For this review, take the finished solid that the model builds, in its own axes (mm). A direction names the side the tool comes from. Round coordinates to 2 decimals unless told otherwise and drop trailing zeros. Loops run counter-clockwise (first coordinate to the right, second up) from the corner with the lowest first, then second, coordinate; pieces in that order, holes last. Notation, with made-up numbers: (11, 36.25) -> (60, 36.25) arc R27 ccw to (60, 62.25) -> close; hole circle Ø10 at (59, 45.25). An arc over 180 degrees is marked (long way). Write each question's results on one line, items separated by ' | '.
```python
from build123d import *

# Parameters (mm, degrees)
Y_KSEKLIK_EKSTR_ZYON1_DEPTH             = 19
IZIM2_W                                 = 40
IZIM2_H                                 = 40
Y_KSEKLIK_EKSTR_ZYON2_DEPTH             = 9
IZIM5_W                                 = 46
IZIM5_H                                 = 46
IZIM5_W_2                               = 40
IZIM5_H_2                               = 40
Y_KSEKLIK_EKSTR_ZYON3_DEPTH             = 9
Y_KSEKLIK_EKSTR_ZYON3_DIRECTION_2_REACH = 172.345
KES_EKSTR_ZYON1_DEPTH                   = 9
KES_EKSTR_ZYON1_DEPTH_BACK              = 9
IZIM7_W                                 = 15
IZIM7_H                                 = 15
IZIM8_R                                 = 3.25
KES_EKSTR_ZYON2_DEPTH                   = 163


with BuildPart() as part:
    # Çizim1 → Yükseklik-Ekstrüzyon1 (new body)
    with BuildSketch(Plane.XY):
        Polygon((0, 0), (0, 80), (133, 80), (133, 0), (138, 0), (138, 30), (142, 30), (142, 89), (-9, 89), (-9, 30), (-5, 30), (-5, 0), align=None)
    extrude(amount=Y_KSEKLIK_EKSTR_ZYON1_DEPTH)

    # Çizim2 → Yükseklik-Ekstrüzyon2 (add)
    with BuildSketch(Plane(origin=(0, 89, 0), x_dir=(1, 0, 0), z_dir=(0, 1, 0))):
        with Locations((66.5, -10.538159249)):
            Rectangle(IZIM2_W, IZIM2_H)
    extrude(amount=-Y_KSEKLIK_EKSTR_ZYON2_DEPTH)

    # Çizim5 → Yükseklik-Ekstrüzyon3 (add)
    with BuildSketch(Plane(origin=(0, 89, 0), x_dir=(1, 0, 0), z_dir=(0, 1, 0))):
        with Locations((66.5, -10.538159249)):
            Rectangle(IZIM5_W, IZIM5_H)
        with Locations((66.5, -10.538159249)):
            Rectangle(IZIM5_W_2, IZIM5_H_2, mode=Mode.SUBTRACT)
    extrude(amount=Y_KSEKLIK_EKSTR_ZYON3_DEPTH)

    # Yükseklik-Ekstrüzyon3 direction 2: up to this face of the body (flat: up to its plane)
    y_kseklik_ekstr_zyon3_direction_2_end = Plane(part.part.faces().sort_by_distance((66.5, 80, 9.993333768))[0])
    # Çizim5 → Yükseklik-Ekstrüzyon3 direction 2 (add, up to the picked face)
    with BuildSketch(Plane(origin=(0, 89, 0), x_dir=(1, 0, 0), z_dir=(0, 1, 0)), mode=Mode.PRIVATE) as y_kseklik_ekstr_zyon3_direction_2_sk1:
        with Locations((66.5, -10.538159249)):
            Rectangle(IZIM5_W, IZIM5_H)
        with Locations((66.5, -10.538159249)):
            Rectangle(IZIM5_W_2, IZIM5_H_2, mode=Mode.SUBTRACT)
    y_kseklik_ekstr_zyon3_direction_2_tool1 = split(extrude(y_kseklik_ekstr_zyon3_direction_2_sk1.sketch, amount=-Y_KSEKLIK_EKSTR_ZYON3_DIRECTION_2_REACH, mode=Mode.PRIVATE), bisect_by=y_kseklik_ekstr_zyon3_direction_2_end, keep=Keep.BOTH, mode=Mode.PRIVATE)
    add(y_kseklik_ekstr_zyon3_direction_2_tool1.solids().sort_by(Axis((66.5, 89, 32.887621), (0, -1, 0)))[0])

    # Çizim7 → Kes-Ekstrüzyon1 (cut, two sides: drawn at the far end of the back side and taken through both)
    with BuildSketch(Plane(origin=(0, 89, 0), x_dir=(1, 0, 0), z_dir=(0, 1, 0)).offset(-KES_EKSTR_ZYON1_DEPTH_BACK)):
        with Locations((66.5, -10.538159249)):
            Rectangle(IZIM7_W, IZIM7_H)
    extrude(amount=KES_EKSTR_ZYON1_DEPTH + KES_EKSTR_ZYON1_DEPTH_BACK, mode=Mode.SUBTRACT)

    # Çizim8 → Kes-Ekstrüzyon2 (cut)
    with BuildSketch(Plane(origin=(138, 0, 0), x_dir=(0, 0, -1), z_dir=(1, 0, 0))):
        with Locations((-9.5, 15)):
            Circle(IZIM8_R)
    extrude(amount=-KES_EKSTR_ZYON2_DEPTH, mode=Mode.SUBTRACT)


solid = part.part
```
1. Consider section C-C (y = 45.5). State the section outline as (x, z) points, plus the area to 3 significant figures.
Values found:
outline: (-9, 0) -> (0, 0) -> (0, 19) -> (-9, 19) -> close; (133, 0) -> (142, 0) -> (142, 19) -> (133, 19) -> close | area: 342 mm2
2. To check wall thickness, follow probe 1 along Y at (x, z) = (137.05, 9.5); probe 2 along X at (y, z) = (49, 9.5); probe 3 along Y at (x, z) = (-0.5, 17.5). State the ranges of each line that lie inside material, in increasing order.
Values found:
probe 1: y = 0 to 11.75, 18.25 to 89 | probe 2: x = -9 to 0, 133 to 142 | probe 3: y = 0 to 89
3. Consider section B-B (y = 90.5). State the section outline as (x, z) points.
Values found:
outline: (43.5, -12.46) -> (89.5, -12.46) -> (89.5, 33.54) -> (43.5, 33.54) -> close; hole (46.5, -9.46) -> (86.5, -9.46) -> (86.5, 30.54) -> (46.5, 30.54) -> close
4. For pin 1 (5 mm diameter, centred on x = 42, z = -7.5, fed in from -Y); pin 2 (4.5 mm diameter, centred on y = 95, z = 2, fed in from -X); pin 3 (8.5 mm diameter, centred on y = 15, z = 9.5, fed in from +X), all flat-tipped, find the tip position at first contact; note any pin that passes through.
Values found:
pin 1: stops at y = 80 | pin 2: stops at x = 43.5 | pin 3: stops at x = 138
5. Consider section A-A (z = 9.5). Give the number of separate pieces and of enclosed holes in the cut face, plus the area to 3 significant figures.
Values found:
separate pieces: 4 | enclosed holes: 0 | area: 2,410 mm2
6. Tool access review of faces 4 (the face through (86.5, 93, 11)), 5 (the face through (-7, 30, 9)), 6 (the face through (17, 89, 9)): name each direction out of +Z, -Z, +X, -X, +Y, -Y from which nothing blocks a thin tool from reaching the whole face with its end or side.
Values found:
face 4: +Y | face 5: +Z, -Z, -X, -Y | face 6: +Z, -Z, -X, +Y
7. Draft analysis for pull direction X (two halves, no side actions). For faces 1 (the face through (138, 11, 9)), 2 (the face through (46.5, 93, 11)), 3 (the face through (-0.4, 61.2, 19)), state which applies: released by +X, released by -X, zero draft, split by the parting line, or undercut.
Values found:
face 1: released by +X | face 2: undercut | face 3: zero draft
8. Consider section D-D (y = 15). State the section outline as (x, z) points, plus the area to 3 significant figures.
Values found:
outline: (-5, 0) -> (0, 0) -> (0, 6.25) -> (-5, 6.25) -> close; (-5, 12.75) -> (0, 12.75) -> (0, 19) -> (-5, 19) -> close; (133, 0) -> (138, 0) -> (138, 6.25) -> (133, 6.25) -> close; (133, 12.75) -> (138, 12.75) -> (138, 19) -> (133, 19) -> close | area: 125 mm2
